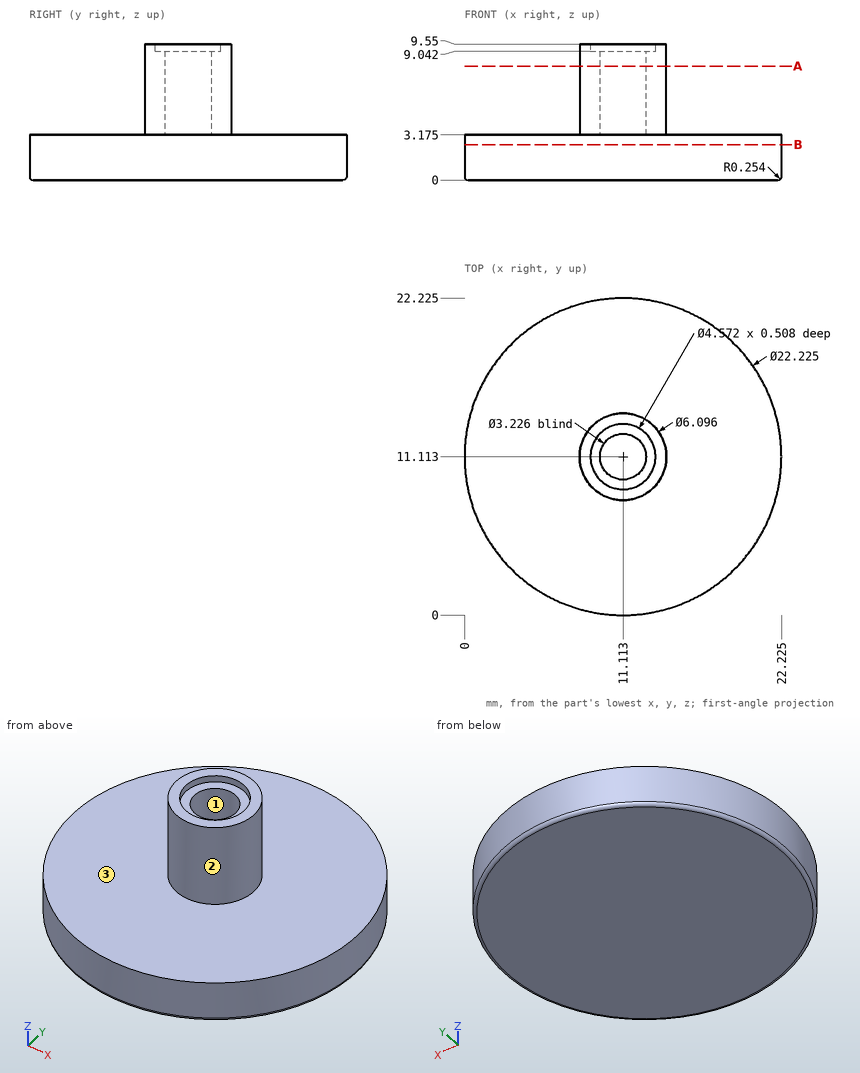
Input: dimensioned drawing with shaded views. Units: mm. Origin: part minimum x, y, z. Coordinates: 2 decimals unless noted, no trailing zeros. Loops run counter-clockwise (first coordinate to the right, second up) from the corner with the lowest first, then second, coordinate; pieces in that order, holes last. Notation, with made-up numbers: M 4.5,-28.5 L 37.5,-28.5 A15 ccw 37.5,0.5 Z; hole C 88.5,89 d4. An arc over 180 degrees is marked long. Use a Markdown table: item, result. Add a question column.
1) Line query: L1, parallel to Z at x = 5.25, y = 20 (1 decimal); L2, parallel to Y at x = 11, z = 2 (1 decimal). Output: solid intervals per line, ascending. Write a range as from..to.
2) Draft query along Y for the marked faces 1, 2 and 3. Return one class per face: +Y half, -Y half, draft (parallel to the pull), parting line (faces both ways), or undercut.
3) Pin query (flat end, axial travel): P1, Ø4, axis at x = 5, y = 15.5, coming from the +Z side (1 decimal); P2, Ø3.5, axis at x = 10.5, y = 10.5, coming from the +Z side; P3, Ø2, axis at x = 9, z = 6.5, coming from the -Y side (1 decimal); P4, Ø1.5, axis at x = 8.5, z = 1, coming from the +Y side. Return the tip coordinate at first contact, or that it passes through.
4) Section B-B, the plane z = 2.5. Return the cut outline in (x, y) (1 decimal).
5) Section A-A, the plane z = 8. Return the cut outline in (x, y) (1 decimal), plus the area to 3 significant figures.
Answer below:
| question | item | result |
|---|---|---|
| 1 | L1 | 0..3.2 |
| 1 | L2 | 0..22.2 |
| 2 | face 1 | undercut |
| 2 | face 2 | parting line |
| 2 | face 3 | draft |
| 3 | P1 | z = 3.2 |
| 3 | P2 | z = 9.55 |
| 3 | P3 | y = 8.3 |
| 3 | P4 | y = 22.07 |
| 4 | outline | C 11.1,11.1 d22.2 |
| 5 | outline | C 11.1,11.1 d6.1; hole C 11.1,11.1 d3.2 |
| 5 | area | 21.0 mm2 |
